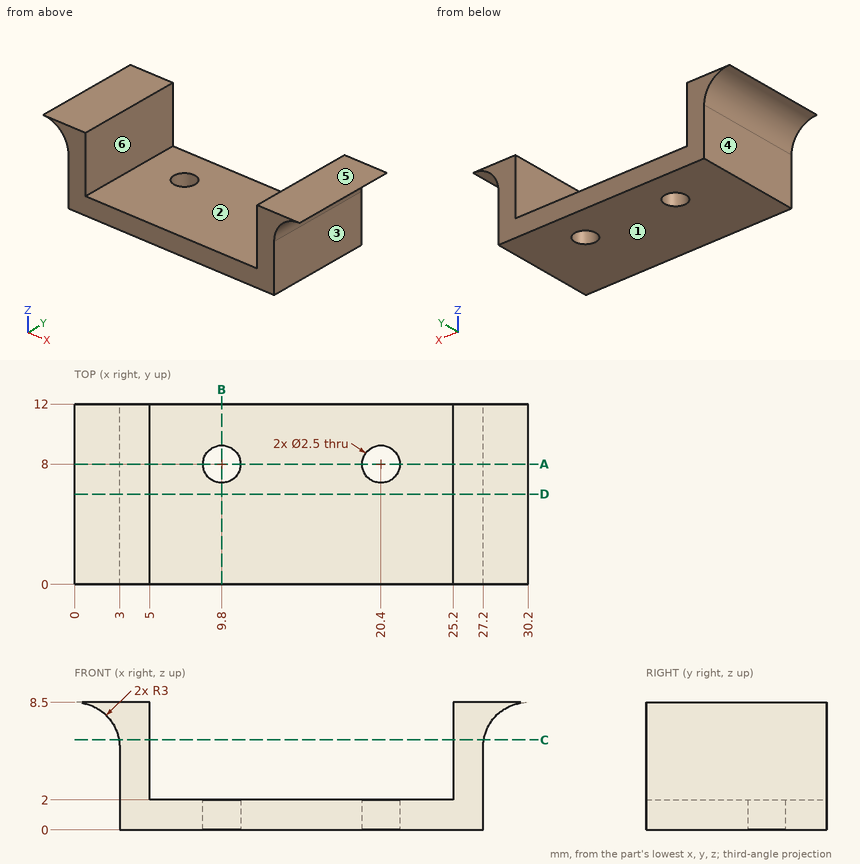
Design review of the part shown in the three views and the two pictorial views. Dimensions are in mm from the part's minimum x, y and z. A direction names the side the tool comes from. Give positions to 0.01 mm unless a question says otherwise; leave off trailing zeros. Loops run counter-clockwise (first coordinate to the right, second up) from the corner with the lowest first, then second, coordinate; pieces in that order, holes last. Notation, with made-up numbers: (11.25, 80) -> (43.25, 80) arc R8 ccw to (43.25, 95) -> close; hole circle Ø4 at (59, -38). An arc over 180 degrees is marked (long way). Answer as a JSON object with one key per item and string values. Group by question number.
Q1. Tool access review of the marked faces 1 and 2: name each direction out of +Z, -Z, +X, -X, +Y, -Y from which nothing blocks a thin tool from reaching the whole face with its end or side.
Q2. Take a section at A-A (y = 8). Write out the cut boundary in (x, z).
Q3. Wall thickness on line 1 along X through (y, z) = (11.5, 4.5); line 2 along Y through (x, z) = (20.4, 1.5); line 3 along X through (y, z) = (7.25, 0.75): over which ranges is each line inside the solid? List them lowest first.
Q4. Insertion check: pin 1 (3 mm diameter, centred on y = 4, z = 4, fed in from +X); pin 2 (4 mm diameter, centred on x = 16, y = 7.5, fed in from +Z); pin 3 (5 mm diameter, centred on y = 8, z = 5, fed in from -X). Each pin has a flat end and moves straight along its axis. Give the tip position at first contact, or say it passes through.
Q5. Draft analysis for pull direction X (two halves, no side actions). For the marked faces 3, 4, 5 and 6, state which applies: pulls with the +X half, pulls with the -X half, needs draft (parallel to the pull), parting line crosses it, or undercut.
Q6. Take a section at C-C (z = 6). Write out the cut boundary in (x, y), plus the area to 3 significant figures.
Q7. Take a section at D-D (y = 6). Write out the cut boundary in (x, z).
Q8. Take a section at B-B (x = 9.8). Write out the cut boundary in (y, z), plus the area to 3 significant figures.
Answer below:
{
 "1": {"face 1": "-Z, +X, -X, +Y, -Y", "face 2": "+Z, +Y, -Y"},
 "2": {"outline": "(0, 8.5) arc R3 cw to (3, 5.5) -> (3, 0) -> (8.55, 0) -> (8.55, 2) -> (5, 2) -> (5, 8.5) -> close; (11.05, 0) -> (19.15, 0) -> (19.15, 2) -> (11.05, 2) -> close; (21.65, 0) -> (27.2, 0) -> (27.2, 5.5) arc R3 cw to (30.2, 8.5) -> (25.2, 8.5) -> (25.2, 2) -> (21.65, 2) -> close"},
 "3": {"line 1": "x = 3 to 5, 25.2 to 27.2", "line 2": "y = 0 to 6.75, 9.25 to 12", "line 3": "x = 3 to 8.8, 10.8 to 19.4, 21.4 to 27.2"},
 "4": {"pin 1": "stops at x = 27.2", "pin 2": "stops at z = 2", "pin 3": "stops at x = 2.24"},
 "5": {"face 3": "pulls with the +X half", "face 4": "pulls with the -X half", "face 5": "needs draft", "face 6": "undercut"},
 "6": {"outline": "(2.96, 0) -> (5, 0) -> (5, 12) -> (2.96, 12) -> close; (25.2, 0) -> (27.24, 0) -> (27.24, 12) -> (25.2, 12) -> close", "area": "49.0 mm2"},
 "7": {"outline": "(0, 8.5) arc R3 cw to (3, 5.5) -> (3, 0) -> (27.2, 0) -> (27.2, 5.5) arc R3 cw to (30.2, 8.5) -> (25.2, 8.5) -> (25.2, 2) -> (5, 2) -> (5, 8.5) -> close"},
 "8": {"outline": "(0, 0) -> (6.75, 0) -> (6.75, 2) -> (0, 2) -> close; (9.25, 0) -> (12, 0) -> (12, 2) -> (9.25, 2) -> close", "area": "19.0 mm2"}
}
